```python
from build123d import *

# Parameters (mm, degrees)
F0_R     = 1
F1_DEPTH = 1.5


with BuildPart() as f1:
    # F0 (on Right) → F1 (new body, symmetric)
    with BuildSketch(Plane.YZ):
        with BuildLine():
            ThreePointArc((55.5, 0), (56.5, 1), (57.5, 0))
            Line((57.5, 0), (58, 0))
            Line((58, 0), (58, 3.5))
            Line((58, 3.5), (55, 3.5))
            Line((55, 3.5), (55, 13.5))
            Line((55, 13.5), (58, 13.5))
            Line((58, 13.5), (58, 20.5))
            Line((58, 20.5), (35, 20.5))
            Line((35, 20.5), (35, 17.5))
            Line((35, 17.5), (25, 17.5))
            Line((25, 17.5), (25, 20.5))
            Line((25, 20.5), (5, 20.5))
            Line((5, 20.5), (5, 17.5))
            Line((5, 17.5), (0, 17.5))
            Line((0, 17.5), (0, 0))
            Line((0, 0), (55.5, 0))
        make_face()
        with Locations((15, 19)):
            Circle(F0_R, mode=Mode.SUBTRACT)
        with BuildLine():
            Line((58, 0), (57.5, 0))
            ThreePointArc((57.5, 0), (56.5, -1), (55.5, 0))
            Line((55.5, 0), (0, 0))
            Line((0, 0), (0, -17.5))
            Line((0, -17.5), (5, -17.5))
            Line((5, -17.5), (5, -20.5))
            Line((5, -20.5), (25, -20.5))
            Line((25, -20.5), (25, -17.5))
            Line((25, -17.5), (35, -17.5))
            Line((35, -17.5), (35, -20.5))
            Line((35, -20.5), (58, -20.5))
            Line((58, -20.5), (58, -13.5))
            Line((58, -13.5), (55, -13.5))
            Line((55, -13.5), (55, -3.5))
            Line((55, -3.5), (58, -3.5))
            Line((58, -3.5), (58, 0))
        make_face()
        with Locations((15, -19)):
            Circle(F0_R, mode=Mode.SUBTRACT)
        with BuildLine():
            Line((-55.5, 0), (0, 0))
            Line((0, 0), (0, 17.5))
            Line((0, 17.5), (-5, 17.5))
            Line((-5, 17.5), (-5, 20.5))
            Line((-5, 20.5), (-25, 20.5))
            Line((-25, 20.5), (-25, 17.5))
            Line((-25, 17.5), (-35, 17.5))
            Line((-35, 17.5), (-35, 20.5))
            Line((-35, 20.5), (-58, 20.5))
            Line((-58, 20.5), (-58, 13.5))
            Line((-58, 13.5), (-55, 13.5))
            Line((-55, 13.5), (-55, 3.5))
            Line((-55, 3.5), (-58, 3.5))
            Line((-58, 3.5), (-58, 0))
            Line((-58, 0), (-57.5, 0))
            ThreePointArc((-57.5, 0), (-56.5, 1), (-55.5, 0))
        make_face()
        with Locations((-15, 19)):
            Circle(F0_R, mode=Mode.SUBTRACT)
        with BuildLine():
            Line((0, -17.5), (0, 0))
            Line((0, 0), (-55.5, 0))
            ThreePointArc((-55.5, 0), (-56.5, -1), (-57.5, 0))
            Line((-57.5, 0), (-58, 0))
            Line((-58, 0), (-58, -3.5))
            Line((-58, -3.5), (-55, -3.5))
            Line((-55, -3.5), (-55, -13.5))
            Line((-55, -13.5), (-58, -13.5))
            Line((-58, -13.5), (-58, -20.5))
            Line((-58, -20.5), (-35, -20.5))
            Line((-35, -20.5), (-35, -17.5))
            Line((-35, -17.5), (-25, -17.5))
            Line((-25, -17.5), (-25, -20.5))
            Line((-25, -20.5), (-5, -20.5))
            Line((-5, -20.5), (-5, -17.5))
            Line((-5, -17.5), (0, -17.5))
        make_face()
        with Locations((-15, -19)):
            Circle(F0_R, mode=Mode.SUBTRACT)
    extrude(amount=F1_DEPTH, both=True)


solid = f1.part
```
Here's how the part is built. I have some questions about the finished solid (model axes, mm). A direction names the side the tool comes from. Give positions to 0.01 mm unless a question says otherwise; leave off trailing zeros. Loops run counter-clockwise (first coordinate to the right, second up) from the corner with the lowest first, then second, coordinate; pieces in that order, holes last. Notation, with made-up numbers: M 83,84 L 105,84 A25 cw 105,111 Z; hole C 26.5,-23.75 d9. An arc over 180 degrees is marked long. Use one line per item in the form item = value. Start each with the question number.
Q1. Which directions (+Z, -Z, +X, -X, +Y, -Y) give clear straight access to the entire face, cutting with the end or side of a thin tool? Please do faces 5 (the flat face through (0, 56, 13.5)), 6 (the flat face through (0, 0, -17.5)), 7 (the flat face through (0, -57, 13.5)), 8 (the flat face through (0, 35, 19)).
Q2. If we section it at A-A (y = 15): Write out the boundary of the cut face in (x, z), then the cut area to 3 significant figures.
Q3. If we section it at D-D (x = -0.7): State how many separate pieces and enclosed holes the cut face has, then the cut area to 3 significant figures.
Q4. If we section it at B-B (z = -19): Write out the boundary of the cut face in (x, y).
Q5. Will this pin go through, and if not, where does the flat tip stop? pin 1 Ø1.5 at (x, y) = (0, 32) entering from +Z.
Q6. I need wall thicknesses on line 1 along Z through (x, y) = (0.8, -15); line 2 along Z through (x, y) = (0.8, 56.5); line 3 along Z through (x, y) = (0.95, -25.5). Which ranges of each line are inside material? Lowest first, please.
Q7. If we section it at C-C (y = 56.5): Write out the boundary of the cut face in (x, z).
Q8. Thinking about a two-plate mould opening in Y: for faces 1 (the flat face through (0, 57, 3.5)), 2 (the flat face through (0, 55, 8)), 3 (the flat face through (0, -30, 17.5)), 4 (the cylindrical face through (0, 15, 18)), which applies, +Y half, -Y half, draft (parallel to the pull), parting line (faces both ways), or undercut?
Taken from the geometry:
q1.face_5 = +X, -X, +Y
q1.face_6 = -Z, +X, -X
q1.face_7 = +X, -X, -Y
q1.face_8 = +Z, +X, -X
q2.outline = M -1.5,-20.5 L 1.5,-20.5 L 1.5,-20 L -1.5,-20 Z; M -1.5,-18 L 1.5,-18 L 1.5,18 L -1.5,18 Z; M -1.5,20 L 1.5,20 L 1.5,20.5 L -1.5,20.5 Z
q2.area = 111 mm^2
q3.separate_pieces = 1
q3.enclosed_holes = 6
q3.area = 4,440 mm^2
q4.outline = M -1.5,-58 L 1.5,-58 L 1.5,-35 L -1.5,-35 Z; M -1.5,-25 L 1.5,-25 L 1.5,-16 L -1.5,-16 Z; M -1.5,-14 L 1.5,-14 L 1.5,-5 L -1.5,-5 Z; M -1.5,5 L 1.5,5 L 1.5,14 L -1.5,14 Z; M -1.5,16 L 1.5,16 L 1.5,25 L -1.5,25 Z; M -1.5,35 L 1.5,35 L 1.5,58 L -1.5,58 Z
q5.pin_1 = 17.5
q6.line_1 = -20.5 to -20, -18 to 18, 20 to 20.5
q6.line_2 = -20.5 to -13.5, -3.5 to -1, 1 to 3.5, 13.5 to 20.5
q6.line_3 = -17.5 to 17.5
q7.outline = M -1.5,-20.5 L 1.5,-20.5 L 1.5,-13.5 L -1.5,-13.5 Z; M -1.5,-3.5 L 1.5,-3.5 L 1.5,-1 L -1.5,-1 Z; M -1.5,1 L 1.5,1 L 1.5,3.5 L -1.5,3.5 Z; M -1.5,13.5 L 1.5,13.5 L 1.5,20.5 L -1.5,20.5 Z
q8.face_1 = draft
q8.face_2 = +Y half
q8.face_3 = undercut
q8.face_4 = undercut
